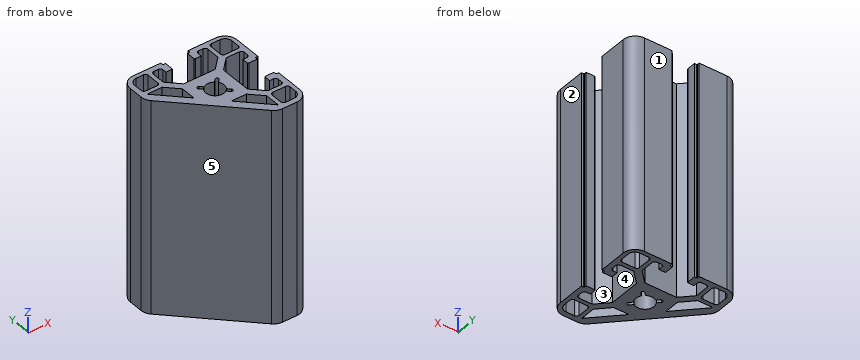
```python
from build123d import *

# Parameters (mm, degrees)
EXTRUDE_1_DEPTH = 80


with BuildPart() as part:
    # 草图1 → 凸台-拉伸1 (new body)
    with BuildSketch(Plane.XY):
        with BuildLine():
            Line((2339.183862097, 210.472909404), (2328.783862097, 210.472909404))
            ThreePointArc((2328.783862097, 210.472909404), (2325.601881582, 209.15488992), (2324.283862097, 205.972909404))
            Line((2324.283862097, 205.972909404), (2324.283862097, 200.621141682))
            ThreePointArc((2324.283862097, 200.621141682), (2324.626404201, 198.899066237), (2325.601881582, 197.439161167))
            Line((2325.601881582, 197.439161167), (2351.25011386, 171.790928889))
            ThreePointArc((2351.25011386, 171.790928889), (2352.71001893, 170.815451508), (2354.432094375, 170.472909404))
            Line((2354.432094375, 170.472909404), (2359.783862097, 170.472909404))
            ThreePointArc((2359.783862097, 170.472909404), (2362.965842612, 171.790928889), (2364.283862097, 174.972909404))
            Line((2364.283862097, 174.972909404), (2364.283862097, 185.372909404))
            Line((2364.283862097, 185.372909404), (2363.483862097, 185.372909404))
            ThreePointArc((2363.483862097, 185.372909404), (2363.342440741, 185.431488048), (2363.283862097, 185.572909404))
            Line((2363.283862097, 185.572909404), (2363.283862097, 186.372909404))
            Line((2363.283862097, 186.372909404), (2360.083862097, 186.372909404))
            ThreePointArc((2360.083862097, 186.372909404), (2359.871730063, 186.285041439), (2359.783862097, 186.072909404))
            Line((2359.783862097, 186.072909404), (2359.783862097, 183.872909404))
            Line((2359.783862097, 183.872909404), (2361.283862097, 183.872909404))
            ThreePointArc((2361.283862097, 183.872909404), (2361.990968878, 183.580016185), (2362.283862097, 182.872909404))
            Line((2362.283862097, 182.872909404), (2362.283862097, 181.222909404))
            ThreePointArc((2362.283862097, 181.222909404), (2361.990968878, 180.515802623), (2361.283862097, 180.222909404))
            Line((2361.283862097, 180.222909404), (2356.30162905, 180.222909404))
            Line((2356.30162905, 180.222909404), (2351.983862097, 184.540676357))
            Line((2351.983862097, 184.540676357), (2351.983862097, 196.405142451))
            Line((2351.983862097, 196.405142451), (2356.30162905, 200.722909404))
            Line((2356.30162905, 200.722909404), (2361.283862097, 200.722909404))
            ThreePointArc((2361.283862097, 200.722909404), (2361.990968878, 200.430016185), (2362.283862097, 199.722909404))
            Line((2362.283862097, 199.722909404), (2362.283862097, 198.072909404))
            ThreePointArc((2362.283862097, 198.072909404), (2361.990968878, 197.365802623), (2361.283862097, 197.072909404))
            Line((2361.283862097, 197.072909404), (2359.783862097, 197.072909404))
            Line((2359.783862097, 197.072909404), (2359.783862097, 194.872909404))
            ThreePointArc((2359.783862097, 194.872909404), (2359.871730063, 194.66077737), (2360.083862097, 194.572909404))
            Line((2360.083862097, 194.572909404), (2363.283862097, 194.572909404))
            Line((2363.283862097, 194.572909404), (2363.283862097, 195.372909404))
            ThreePointArc((2363.283862097, 195.372909404), (2363.342440741, 195.514330761), (2363.483862097, 195.572909404))
            Line((2363.483862097, 195.572909404), (2364.283862097, 195.572909404))
            Line((2364.283862097, 195.572909404), (2364.283862097, 205.972909404))
            ThreePointArc((2364.283862097, 205.972909404), (2362.965842612, 209.15488992), (2359.783862097, 210.472909404))
            Line((2359.783862097, 210.472909404), (2349.383862097, 210.472909404))
            Line((2349.383862097, 210.472909404), (2349.383862097, 209.672909404))
            ThreePointArc((2349.383862097, 209.672909404), (2349.325283453, 209.531488048), (2349.183862097, 209.472909404))
            Line((2349.183862097, 209.472909404), (2348.383862097, 209.472909404))
            Line((2348.383862097, 209.472909404), (2348.383862097, 206.272909404))
            ThreePointArc((2348.383862097, 206.272909404), (2348.471730063, 206.06077737), (2348.683862097, 205.972909404))
            Line((2348.683862097, 205.972909404), (2350.883862097, 205.972909404))
            Line((2350.883862097, 205.972909404), (2350.883862097, 207.472909404))
            ThreePointArc((2350.883862097, 207.472909404), (2351.176755316, 208.180016185), (2351.883862097, 208.472909404))
            Line((2351.883862097, 208.472909404), (2353.533862097, 208.472909404))
            ThreePointArc((2353.533862097, 208.472909404), (2354.240968878, 208.180016185), (2354.533862097, 207.472909404))
            Line((2354.533862097, 207.472909404), (2354.533862097, 202.490676357))
            Line((2354.533862097, 202.490676357), (2350.216095144, 198.172909404))
            Line((2350.216095144, 198.172909404), (2338.35162905, 198.172909404))
            Line((2338.35162905, 198.172909404), (2334.033862097, 202.490676357))
            Line((2334.033862097, 202.490676357), (2334.033862097, 207.472909404))
            ThreePointArc((2334.033862097, 207.472909404), (2334.326755316, 208.180016185), (2335.033862097, 208.472909404))
            Line((2335.033862097, 208.472909404), (2336.683862097, 208.472909404))
            ThreePointArc((2336.683862097, 208.472909404), (2337.390968878, 208.180016185), (2337.683862097, 207.472909404))
            Line((2337.683862097, 207.472909404), (2337.683862097, 205.972909404))
            Line((2337.683862097, 205.972909404), (2339.883862097, 205.972909404))
            ThreePointArc((2339.883862097, 205.972909404), (2340.095994131, 206.06077737), (2340.183862097, 206.272909404))
            Line((2340.183862097, 206.272909404), (2340.183862097, 209.472909404))
            Line((2340.183862097, 209.472909404), (2339.383862097, 209.472909404))
            ThreePointArc((2339.383862097, 209.472909404), (2339.242440741, 209.531488048), (2339.183862097, 209.672909404))
            Line((2339.183862097, 209.672909404), (2339.183862097, 210.472909404))
        make_face()
        with BuildLine():
            Line((2326.279862097, 206.476909404), (2326.279862097, 203.222909404))
            ThreePointArc((2326.279862097, 203.222909404), (2326.572755316, 202.515802623), (2327.279862097, 202.222909404))
            Line((2327.279862097, 202.222909404), (2331.533862097, 202.222909404))
            ThreePointArc((2331.533862097, 202.222909404), (2332.240968878, 202.515802623), (2332.533862097, 203.222909404))
            Line((2332.533862097, 203.222909404), (2332.533862097, 207.976909404))
            ThreePointArc((2332.533862097, 207.976909404), (2332.240968878, 208.684016185), (2331.533862097, 208.976909404))
            Line((2331.533862097, 208.976909404), (2328.779862097, 208.976909404))
            ThreePointArc((2328.779862097, 208.976909404), (2327.012095144, 208.244676357), (2326.279862097, 206.476909404))
        make_face(mode=Mode.SUBTRACT)
        Polygon((2344.510774032, 182.772909404), (2350.216095144, 182.772909404), (2354.533862097, 178.455142451), (2354.533862097, 172.749821339), align=None, mode=Mode.SUBTRACT)
        Polygon((2336.583862097, 196.405142451), (2336.583862097, 190.699821339), (2326.560774032, 200.722909404), (2332.266095144, 200.722909404), align=None, mode=Mode.SUBTRACT)
        with BuildLine():
            Line((2362.787862097, 206.476909404), (2362.787862097, 203.222909404))
            ThreePointArc((2362.787862097, 203.222909404), (2362.494968878, 202.515802623), (2361.787862097, 202.222909404))
            Line((2361.787862097, 202.222909404), (2357.033862097, 202.222909404))
            ThreePointArc((2357.033862097, 202.222909404), (2356.326755316, 202.515802623), (2356.033862097, 203.222909404))
            Line((2356.033862097, 203.222909404), (2356.033862097, 207.976909404))
            ThreePointArc((2356.033862097, 207.976909404), (2356.326755316, 208.684016185), (2357.033862097, 208.976909404))
            Line((2357.033862097, 208.976909404), (2360.287862097, 208.976909404))
            ThreePointArc((2360.287862097, 208.976909404), (2362.05562905, 208.244676357), (2362.787862097, 206.476909404))
        make_face(mode=Mode.SUBTRACT)
        with BuildLine():
            Line((2362.787862097, 174.968909404), (2362.787862097, 177.722909404))
            ThreePointArc((2362.787862097, 177.722909404), (2362.494968878, 178.430016185), (2361.787862097, 178.722909404))
            Line((2361.787862097, 178.722909404), (2357.033862097, 178.722909404))
            ThreePointArc((2357.033862097, 178.722909404), (2356.326755316, 178.430016185), (2356.033862097, 177.722909404))
            Line((2356.033862097, 177.722909404), (2356.033862097, 173.468909404))
            ThreePointArc((2356.033862097, 173.468909404), (2356.326755316, 172.761802623), (2357.033862097, 172.468909404))
            Line((2357.033862097, 172.468909404), (2360.287862097, 172.468909404))
            ThreePointArc((2360.287862097, 172.468909404), (2362.05562905, 173.201142451), (2362.787862097, 174.968909404))
        make_face(mode=Mode.SUBTRACT)
        with BuildLine():
            Line((2347.324421256, 194.361996701), (2346.226029942, 193.263605386))
            ThreePointArc((2346.226029942, 193.263605386), (2344.283862097, 193.872909404), (2342.341694253, 193.263605386))
            Line((2342.341694253, 193.263605386), (2341.243302938, 194.361996701))
            ThreePointArc((2341.243302938, 194.361996701), (2340.394774801, 194.361996701), (2340.394774801, 193.513468563))
            Line((2340.394774801, 193.513468563), (2341.493166115, 192.415077249))
            ThreePointArc((2341.493166115, 192.415077249), (2341.879699041, 188.068746348), (2346.226029942, 187.682213422))
            Line((2346.226029942, 187.682213422), (2347.324421256, 186.583822108))
            ThreePointArc((2347.324421256, 186.583822108), (2348.172949394, 186.583822108), (2348.172949394, 187.432350245))
            Line((2348.172949394, 187.432350245), (2347.074558079, 188.53074156))
            ThreePointArc((2347.074558079, 188.53074156), (2347.683862097, 190.472909404), (2347.074558079, 192.415077249))
            Line((2347.074558079, 192.415077249), (2348.172949394, 193.513468563))
            ThreePointArc((2348.172949394, 193.513468563), (2348.172949394, 194.361996701), (2347.324421256, 194.361996701))
        make_face(mode=Mode.SUBTRACT)
    extrude(amount=EXTRUDE_1_DEPTH)


solid = part.part
```
Work out the finished part from the listing and answer in its coordinate system (mm). Face numbers are marked on the shaded views. A direction names the side the tool comes from. Give positions to 0.01 mm unless a question says otherwise; leave off trailing zeros. Loops run counter-clockwise (first coordinate to the right, second up) from the corner with the lowest first, then second, coordinate; pieces in that order, holes last. Notation, with made-up numbers: (-27, -32) -> (15, -32) arc R22 ccw to (15, -18) -> close; hole circle Ø9 at (54, 45.5). An arc over 180 degrees is marked (long way). Use CSV: the item, a comma, the result in double quotes.
1. Flat-ended cylindrical pins translate along their axes: pin 1 Ø5 at (y, z) = (177.5, 71.5) entering from -X; pin 2 Ø0.7 at (y, z) = (184.5, 30.5) entering from -X; pin 3 Ø4 at (y, z) = (185, 68) entering from -X. Find the tip coordinate at first contact, or state that the pin passes through.
Found:
pin 1,"x = 2343.04"
pin 2,"x = 2338.19"
pin 3,"x = 2336.04"
2. Straight lines are drawn through the part: line 1 (X direction, y = 205, z = 22); line 2 (X direction, y = 177.5, z = 27); line 3 (Y direction, x = 2357, z = 39.5). For each, find the intervals that lie inside material, in ascending order.
Found:
line 1,"2324.28 to 2326.28, 2332.53 to 2334.03, 2354.53 to 2356.03, 2362.79 to 2364.28"
line 2,"2345.54 to 2349.78, 2354.53 to 2356.03, 2362.79 to 2364.28"
line 3,"170.47 to 172.47, 178.72 to 180.22, 200.72 to 202.22, 208.98 to 210.47"
3. The part is cut by section A-A (y = 205). Write down the section's boundary in (x, z).
Found:
outline,"(2324.28, 0) -> (2326.28, 0) -> (2326.28, 80) -> (2324.28, 80) -> close; (2332.53, 0) -> (2334.03, 0) -> (2334.03, 80) -> (2332.53, 80) -> close; (2354.53, 0) -> (2356.03, 0) -> (2356.03, 80) -> (2354.53, 80) -> close; (2362.79, 0) -> (2364.28, 0) -> (2364.28, 80) -> (2362.79, 80) -> close"
4. The mould has two halves that part along Y. Classify the marked faces 1, 2 and 3: +Y half, -Y half, draft (parallel to the pull), parting line (faces both ways), or undercut.
Found:
face 1,"+Y half"
face 2,"draft"
face 3,"undercut"
5. A tool of negligible diameter and unlimited length cuts with its end or side. For the marked faces 4 and 5, from which of +Z, -Z, +X, -X, +Y, -Y can it reach the whole face along a straight path? Write none if from no direction.
Found:
face 4,"+Z, -Z"
face 5,"+Z, -Z, -X, -Y"
6. The part is cut by section C-C (z = 69.5). State how many separate pieces and enclosed holes the cut face has, then the cut area to 3 significant figures.
Found:
separate pieces,"1"
enclosed holes,"6"
area,"542 mm^2"
7. The part is cut by section B-B (y = 189.5). Write down the section's boundary in (x, z).
Found:
outline,"(2333.54, 0) -> (2341.03, 0) -> (2341.03, 80) -> (2333.54, 80) -> close; (2347.54, 0) -> (2351.98, 0) -> (2351.98, 80) -> (2347.54, 80) -> close"
